```python
from build123d import *

# Parameters (mm, degrees)
CROQUIS1_W              = 60
CROQUIS1_H              = 15
CROQUIS1_R              = 3
SALIENTE_EXTRUIR1_DEPTH = 11
REDONDEO1_R             = 5
CORTAR_EXTRUIR1_DEPTH   = 21
CHAFL_N1_SIZE           = 1


with BuildPart() as part:
    # Croquis1 → Saliente-Extruir1 (new body)
    with BuildSketch(Plane.XY):
        with Locations((30, 7.5)):
            Rectangle(CROQUIS1_W, CROQUIS1_H)
        with Locations((5, 7.5)):
            Circle(CROQUIS1_R, mode=Mode.SUBTRACT)
        with Locations((55, 7.5)):
            Circle(CROQUIS1_R, mode=Mode.SUBTRACT)
    extrude(amount=SALIENTE_EXTRUIR1_DEPTH)

    # Redondeo1
    redondeo1_edges = [part.edges().sort_by_distance(p)[0] for p in [
        (0, 0, 5.5),
        (0, 15, 5.5),
        (60, 15, 5.5),
        (60, 0, 5.5),
    ]]
    fillet(redondeo1_edges, radius=REDONDEO1_R)

    # Croquis2 → Cortar-Extruir1 (cut)
    with BuildSketch(Plane(origin=(0, 15, 0), x_dir=(1, 0, 0), z_dir=(0, 1, 0))):
        Polygon((30, -11), (48, -11), (48, -6), (12, -6), (12, -11), align=None)
    extrude(amount=-CORTAR_EXTRUIR1_DEPTH, mode=Mode.SUBTRACT)

    # Chaflán1
    chafl_n1_edges = [part.edges().sort_by_distance(p)[0] for p in [
        (2, 7.5, 11),
        (52, 7.5, 11),
    ]]
    chamfer(chafl_n1_edges, length=CHAFL_N1_SIZE)


solid = part.part
```
Could you check a few things on this model? Use its own coordinates, in mm. A direction names the side the tool comes from. Give positions to 0.01 mm unless a question says otherwise; leave off trailing zeros. Order: outer loops, then holes, each group sorted by start corner. A loop starts at its lowest first (then second) coordinate and runs counter-clockwise, first axis right, second up.
Q1. I'm going to push a flat-ended pin straight in: P1, Ø4.5, axis at x = 37, y = 6.5, coming from the +Z side. Where does the tip first touch, or does it pass through?
Q2. We'd pull the mould along X, two halves only. Please class faces 3 (the cylindrical face through (52, 7.6, 4.9)), 4 (the flat face through (60, 7, 5)), 5 (the flat face through (30, 0, 4)): +X half, -X half, draft (parallel to the pull), parting line (faces both ways), or undercut.
Q3. Suppose I cut it at B-B, the plane y = 13. Write out the boundary of the cut face in (x, z), and give its area (3 significant figures).
Q4. Suppose I cut it at C-C, the plane x = 38.5. Write out the boundary of the cut face in (y, z).
Q5. If I drill on line 1 along X through (y, z) = (6.75, 5.75); line 2 along X through (y, z) = (6, 7.5); line 3 along Y through (x, z) = (55, 6.5), over which ranges is the centre line in solid material (lowest first)?
Q6. Suppose I cut it at A-A, the plane y = 7.5. Write out the boundary of the cut face in (x, z), and give its area (3 significant figures).
Q7. For faces 1 (the flat face through (12, 8, 8)), 2 (the cylindrical face through (1, 2, 6)), which set-ups out of +Z, -Z, +X, -X, +Y, -Y let a thin tool reach every point of the face, with its end or its side?
Solution:
1. P1: stops at z = 6
2. face 3: undercut
2. face 4: +X half
2. face 5: draft
3. outline: (1, 0) - (59, 0) - (59, 11) - (48, 11) - (48, 6) - (12, 6) - (12, 11) - (1, 11) - close
3. area: 458 mm2
4. outline: (0, 0) - (15, 0) - (15, 6) - (0, 6) - close
5. line 1: x = 0 to 2.1, 7.9 to 52.1, 57.9 to 60
5. line 2: x = 0 to 2.4, 7.6 to 12, 48 to 52.4, 57.6 to 60
5. line 3: y = 0 to 4.5, 10.5 to 15
6. outline: (0, 0) - (2, 0) - (2, 10) - (1, 11) - (0, 11) - close; (8, 0) - (52, 0) - (52, 10) - (51, 11) - (48, 11) - (48, 6) - (12, 6) - (12, 11) - (9, 11) - (8, 10) - close; (58, 0) - (60, 0) - (60, 11) - (59, 11) - (58, 10) - close
6. area: 346 mm2
7. face 1: +Z, +Y, -Y
7. face 2: +Z, -Z, -X, -Y
